Study the drawing (mm; zero at the part's minimum x, y, z) and answer. Round coordinates to 2 decimals unless told otherwise and drop trailing zeros. Write each loop counter-clockwise with the first axis right and the second up, starting at its lowest first coordinate (ties: lowest second). Pieces come first, ordered by that corner, then holes.
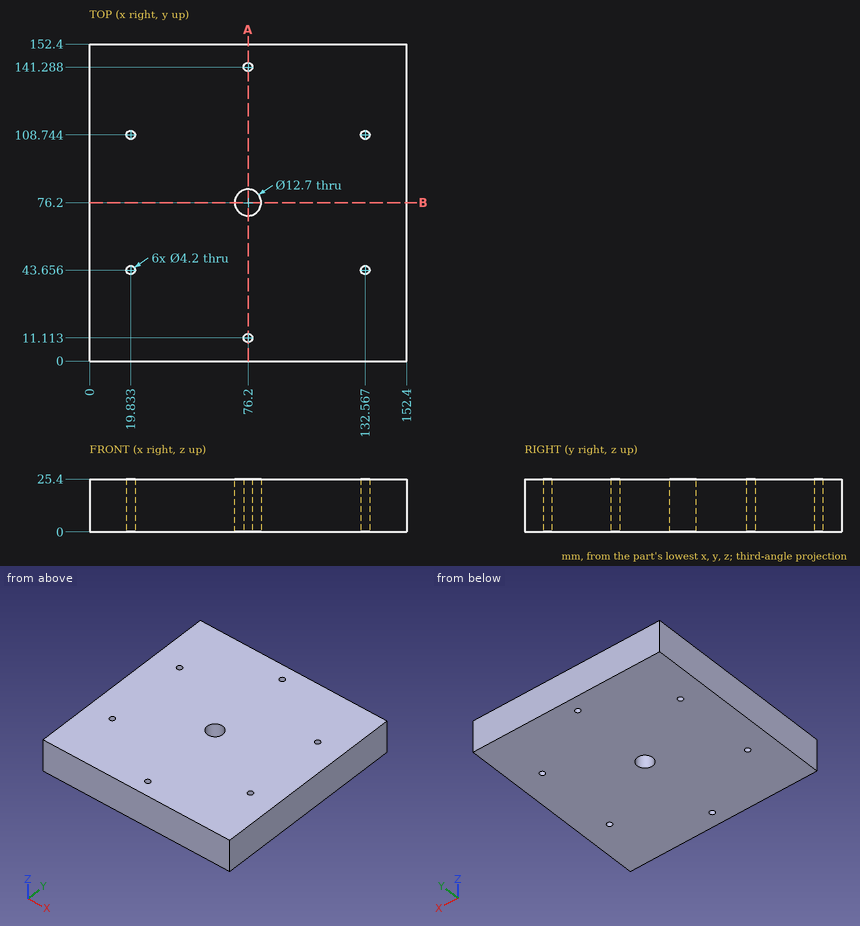
1. Section A-A on x = 76.2 is taken. Determine the outline of the cut face in (y, z), plus the area to 4 significant figures.
Geometry says:
outline: (0, 0) - (9.01, 0) - (9.01, 25.4) - (0, 25.4) - close; (13.21, 0) - (69.85, 0) - (69.85, 25.4) - (13.21, 25.4) - close; (82.55, 0) - (139.19, 0) - (139.19, 25.4) - (82.55, 25.4) - close; (143.39, 0) - (152.4, 0) - (152.4, 25.4) - (143.39, 25.4) - close
area: 3,335 mm2
2. Straight lines are drawn through the part: line 1 along Y through (x, z) = (76.2, 8); line 2 along X through (y, z) = (141, 1.5); line 3 along X through (y, z) = (9.5, 23) (1 decimal). For each, find the intervals that lie inside material, in ascending order.
Geometry says:
line 1: y = 0 to 9.01, 13.21 to 69.85, 82.55 to 139.19, 143.39 to 152.4
line 2: x = 0 to 74.12, 78.28 to 152.4
line 3: x = 0 to 74.9, 77.5 to 152.4
3. Section B-B on y = 76.2 is taken. Determine the outline of the cut face in (x, z).
Geometry says:
outline: (0, 0) - (69.85, 0) - (69.85, 25.4) - (0, 25.4) - close; (82.55, 0) - (152.4, 0) - (152.4, 25.4) - (82.55, 25.4) - close
